Source: CAD feature listing. Evaluate the final solid. Frame: model axes, mm. A direction names the side the tool comes from. Give positions to 0.01 mm unless a question says otherwise; leave off trailing zeros. Loops run counter-clockwise (first coordinate to the right, second up) from the corner with the lowest first, then second, coordinate; pieces in that order, holes last. Notation, with made-up numbers: (26, 87.25) -> (34, 87.25) arc R23 ccw to (34, 95.25) -> close; hole circle Ø10 at (-10, -5). An arc over 180 degrees is marked (long way). Return JSON: item names as keys, results as strings. Group by question number.
(1) Draft query along X for faces 4 (the face through (-172, 11, -105)), 5 (the face through (-204.5, 5, -47)), 6 (the face through (-189.543, 5.577, -48.151)). Return one class per face: released by +X, released by -X, zero draft, split by the parting line, or undercut.
(2) Pin query (flat end, axial travel): pin 1 (5.5 mm diameter, centred on x = -163, y = 25, fed in from +Z); pin 2 (9 mm diameter, centred on y = 4.5, z = -108.5, fed in from +X); pin 3 (6 mm diameter, centred on x = -197.5, z = -45.5, fed in from +Y). Return the tip coordinate at first contact, or that it passes through.
(3) Cut plane A-A on x = -177.5. Return loops of the section in (y, z).
(4) Access query for faces 1 (the face through (-194, 6, -60)), 2 (the face through (-161, 19, -84)), 3 (the face through (-189.9, 11, -50.1)). Directions: +Z, -Z, +X, -X, +Y, -Y. A direction counts if a zero-diameter tool reaches every point of the face in a straight line with its end or side. Return the directions, or none.
(5) Cut plane D-D on x = -167.5. Return loops of the section in (y, z), then the cut area to 3 significant figures.
(6) Ray query, line 1 (X direction, y = 6, z = -47.5); line 2 (X direction, y = 7.25, z = -110); line 3 (X direction, y = 8.75, z = -73). Return the intervals inside material, ascending. Write a range as from..to.
(7) Cut plane B-B on z = -47.5. Return loops of the section in (x, y).
(8) Cut plane C-C on y = 6.75. Return loops of the section in (x, z), then the cut area to 3 significant figures.
```python
from build123d import *

# Parameters (mm, degrees)
SKETCH1_W               = 369
SKETCH1_H               = 200
BOSS_EXTRUDE1_DEPTH     = 20
SKETCH2_W               = 129
SKETCH2_H               = 16
BOSS_EXTRUDE2_DEPTH     = 10
SKETCH3_W               = 342
SKETCH3_H               = 168
CUT_EXTRUDE1_DEPTH      = 9
SKETCH4_W               = 100
SKETCH4_H               = 10
BOSS_EXTRUDE3_DEPTH     = 60
CUT_EXTRUDE3_DEPTH      = 10
CUT_EXTRUDE3_DEPTH_BACK = 60
SKETCH10_W              = 404
SKETCH10_H              = 324.796202869
CUT_EXTRUDE4_DEPTH      = 69
CUT_EXTRUDE7_DEPTH      = 274.752168941
CUT_EXTRUDE7_DEPTH_BACK = 274.752168941
SKETCH14_W              = 37
SKETCH14_H              = 34.717467541
SKETCH12_W              = 50
SKETCH12_H              = 11
BOSS_EXTRUDE6_DEPTH     = 20
SKETCH13_R              = 4
CUT_EXTRUDE6_DEPTH      = 229.43215623
CORTAR_EXTRUIR4_DEPTH   = 220
CROQUIS5_W              = 20
CROQUIS5_H              = 11
SALIENTE_EXTRUIR2_DEPTH = 10
CROQUIS6_W              = 20
CROQUIS6_H              = 11
SALIENTE_EXTRUIR3_DEPTH = 20
CROQUIS8_R              = 5
CORTAR_EXTRUIR5_DEPTH   = 48
CROQUIS9_W              = 38
CROQUIS9_H              = 65
CORTAR_EXTRUIR6_DEPTH   = 85


with BuildPart() as part:
    # Sketch1 → Boss-Extrude1 (new body)
    with BuildSketch(Plane(origin=(0, 0, 0), x_dir=(1, 0, 0), z_dir=(0, 1, 0))):
        Rectangle(SKETCH1_W, SKETCH1_H)
    extrude(amount=BOSS_EXTRUDE1_DEPTH)

    # Sketch2 → Boss-Extrude2 (add)
    with BuildSketch(Plane(origin=(0, 20, 0), x_dir=(1, 0, 0), z_dir=(0, 1, 0))):
        Polygon((-184.5, -100), (-169.5, -100), (-119.5, -100), (-119.5, -84), (-169.5, -84), (-169.5, -35), (-184.5, -35), align=None)
        Polygon((-184.5, 100), (-169.5, 100), (-119.5, 100), (-119.5, 84), (-169.5, 84), (-169.5, 35), (-184.5, 35), align=None)
        with Locations((20, -92)):
            Rectangle(SKETCH2_W, SKETCH2_H)
        with Locations((20, 92)):
            Rectangle(SKETCH2_W, SKETCH2_H)
    extrude(amount=BOSS_EXTRUDE2_DEPTH)

    # Sketch3 → Cut-Extrude1 (cut)
    with BuildSketch(Plane(origin=(0, 20, 0), x_dir=(1, 0, 0), z_dir=(0, 1, 0))):
        with Locations((1.5, 0)):
            Rectangle(SKETCH3_W, SKETCH3_H)
    extrude(amount=-CUT_EXTRUDE1_DEPTH, mode=Mode.SUBTRACT)

    # Sketch4 → Boss-Extrude3 (add)
    with BuildSketch(Plane(origin=(0, 0, -100), x_dir=(-1, 0, 0), z_dir=(0, 0, -1))):
        with Locations((-19.5, 25)):
            Rectangle(SKETCH4_W, SKETCH4_H)
    extrude(amount=BOSS_EXTRUDE3_DEPTH)

    # Sketch6 → Cut-Extrude3 (cut, two sides: drawn at the far end of the back side and taken through both)
    with BuildSketch(Plane.XY.offset(-84).offset(-CUT_EXTRUDE3_DEPTH_BACK)):
        with BuildLine():
            Line((-24.5, 30), (-26.030765637, 28.081051534))
            ThreePointArc((-26.030765637, 28.081051534), (-26.158442873, 26.948989892), (-25.193843525, 26.342843758))
            Line((-25.193843525, 26.342843758), (-15.806155854, 26.342843758))
            ThreePointArc((-15.806155854, 26.342843758), (-14.841556992, 26.948990172), (-14.969234363, 28.081051534))
            Line((-14.969234363, 28.081051534), (-16.5, 30))
            Line((-16.5, 30), (-24.5, 30))
        make_face()
        with BuildLine():
            Line((56.5, 30), (54.981983491, 27.801494438))
            ThreePointArc((54.981983491, 27.801494438), (54.9192914, 26.767046688), (55.80615587, 26.230871478))
            Line((55.80615587, 26.230871478), (65.193843541, 26.230871478))
            ThreePointArc((65.193843541, 26.230871478), (66.080708464, 26.767046428), (66.018016509, 27.801494438))
            Line((66.018016509, 27.801494438), (64.5, 30))
            Line((64.5, 30), (56.5, 30))
        make_face()
    extrude(amount=CUT_EXTRUDE3_DEPTH + CUT_EXTRUDE3_DEPTH_BACK, mode=Mode.SUBTRACT)

    # Sketch10 → Cut-Extrude4 (cut)
    with BuildSketch(Plane(origin=(0, 30, 0), x_dir=(1, 0, 0), z_dir=(0, 1, 0))):
        with Locations((55.5, -0.89352463)):
            Rectangle(SKETCH10_W, SKETCH10_H)
    extrude(amount=-CUT_EXTRUDE4_DEPTH, mode=Mode.SUBTRACT)

    # Sketch14 → Cut-Extrude7 (cut, two sides: drawn at the far end of the back side and taken through both)
    with BuildSketch(Plane(origin=(0, 0, -100), x_dir=(-1, 0, 0), z_dir=(0, 0, -1)).offset(-CUT_EXTRUDE7_DEPTH_BACK)):
        with Locations((138, 36.253686327)):
            Rectangle(SKETCH14_W, SKETCH14_H)
    extrude(amount=CUT_EXTRUDE7_DEPTH + CUT_EXTRUDE7_DEPTH_BACK, mode=Mode.SUBTRACT)

    # Sketch12 → Boss-Extrude6 (add)
    with BuildSketch(Plane.ZY.offset(184.5)):
        with Locations((-25, 5.5)):
            Rectangle(SKETCH12_W, SKETCH12_H)
    extrude(amount=BOSS_EXTRUDE6_DEPTH)

    # Sketch13 → Cut-Extrude6 (cut, through all)
    with BuildSketch(Plane(origin=(0, 11, 0), x_dir=(1, 0, 0), z_dir=(0, 1, 0))):
        with Locations(Location((-194.5, 25, 0), (0, 0, 270))):
            Circle(SKETCH13_R)
    extrude(amount=-CUT_EXTRUDE6_DEPTH, mode=Mode.SUBTRACT)

    # Croquis3 → Cortar-Extruir4 (cut)
    with BuildSketch(Plane(origin=(0, 30, 0), x_dir=(1, 0, 0), z_dir=(0, 1, 0))):
        Polygon((-169.5, -35), (-146.5, -35), (-146.5, 0), (-146.5, 35), (-204.5, 35), (-204.5, 0), (-204.5, -35), (-184.5, -35), align=None)
    extrude(amount=-CORTAR_EXTRUIR4_DEPTH, mode=Mode.SUBTRACT)


with BuildPart() as cortar_extruir4_piece_1:
    # of the separate pieces the step leaves, piece 1, a body of its own (cortar_extruir4_pieces)
    add(part.part.solids().sort_by_distance((-184.5, 30, -100))[0])

    # Croquis5 → Saliente-Extruir2 (add)
    with BuildSketch(Plane(origin=(0, 0, -50), x_dir=(-1, 0, 0), z_dir=(0, 0, -1))):
        with Locations((194.5, 5.5)):
            Rectangle(CROQUIS5_W, CROQUIS5_H)
    extrude(amount=SALIENTE_EXTRUIR2_DEPTH)

    # Croquis6 → Saliente-Extruir3 (add)
    with BuildSketch(Plane(origin=(0, 0, -100), x_dir=(-1, 0, 0), z_dir=(0, 0, -1))):
        with Locations((174.5, 5.5)):
            Rectangle(CROQUIS6_W, CROQUIS6_H)
    extrude(amount=SALIENTE_EXTRUIR3_DEPTH)

    # Croquis8 → Cortar-Extruir5 (cut)
    with BuildSketch(Plane(origin=(0, 11, 0), x_dir=(1, 0, 0), z_dir=(0, 1, 0))):
        with Locations(Location((-194.5, 47.5, 0), (0, 0, 270))):
            Circle(CROQUIS8_R)
        with Locations((-194.5, -47.5)):
            Circle(CROQUIS8_R)
        with Locations((-174.5, -110)):
            Circle(CROQUIS8_R)
        with Locations(Location((-174.5, 110, 0), (0, 0, 270))):
            Circle(CROQUIS8_R)
    extrude(amount=-CORTAR_EXTRUIR5_DEPTH, mode=Mode.SUBTRACT)


with BuildPart() as cortar_extruir4_piece_2:
    # of the separate pieces the step leaves, piece 2, a body of its own (cortar_extruir4_pieces)
    add(part.part.solids().sort_by_distance((-184.5, 30, 100))[0])

    # Croquis9 → Cortar-Extruir6 (cut)
    with BuildSketch(Plane(origin=(0, 30, 0), x_dir=(1, 0, 0), z_dir=(0, 1, 0))):
        with Locations((-165.5, -67.5)):
            Rectangle(CROQUIS9_W, CROQUIS9_H)
    extrude(amount=-CORTAR_EXTRUIR6_DEPTH, mode=Mode.SUBTRACT)


solid = cortar_extruir4_piece_1.part
```
Answers:
{
 "1": {"face 4": "zero draft", "face 5": "released by -X", "face 6": "undercut"},
 "2": {"pin 1": "z = -84", "pin 2": "x = -164.5", "pin 3": "y = 11"},
 "3": {"outline": "(0, -120) -> (11, -120) -> (11, -114) -> (0, -114) -> close; (0, -106) -> (11, -106) -> (11, -100) -> (30, -100) -> (30, -35) -> (0, -35) -> close"},
 "4": {"face 1": "-Z, -X, +Y, -Y", "face 2": "+Z, +X, +Y", "face 3": "+Z, -Z, -X, +Y"},
 "5": {"outline": "(0, -120) -> (11, -120) -> (11, -100) -> (30, -100) -> (30, -84) -> (11, -84) -> (11, -35) -> (0, -35) -> close", "area": "1,240 mm²"},
 "6": {"line 1": "-204.5..-199.5, -189.5..-146.5", "line 2": "-184.5..-179.5, -169.5..-164.5", "line 3": "-184.5..-146.5"},
 "7": {"outline": "(-204.5, 0) -> (-199.5, 0) -> (-199.5, 11) -> (-204.5, 11) -> close; (-189.5, 0) -> (-146.5, 0) -> (-146.5, 11) -> (-169.5, 11) -> (-169.5, 30) -> (-184.5, 30) -> (-184.5, 11) -> (-189.5, 11) -> close"},
 "8": {"outline": "(-204.5, -60) -> (-184.5, -60) -> (-184.5, -120) -> (-164.5, -120) -> (-164.5, -100) -> (-146.5, -100) -> (-146.5, -35) -> (-204.5, -35) -> close; hole circle Ø10 at (-194.5, -47.5); hole circle Ø10 at (-174.5, -110)", "area": "3,210 mm²"}
}
